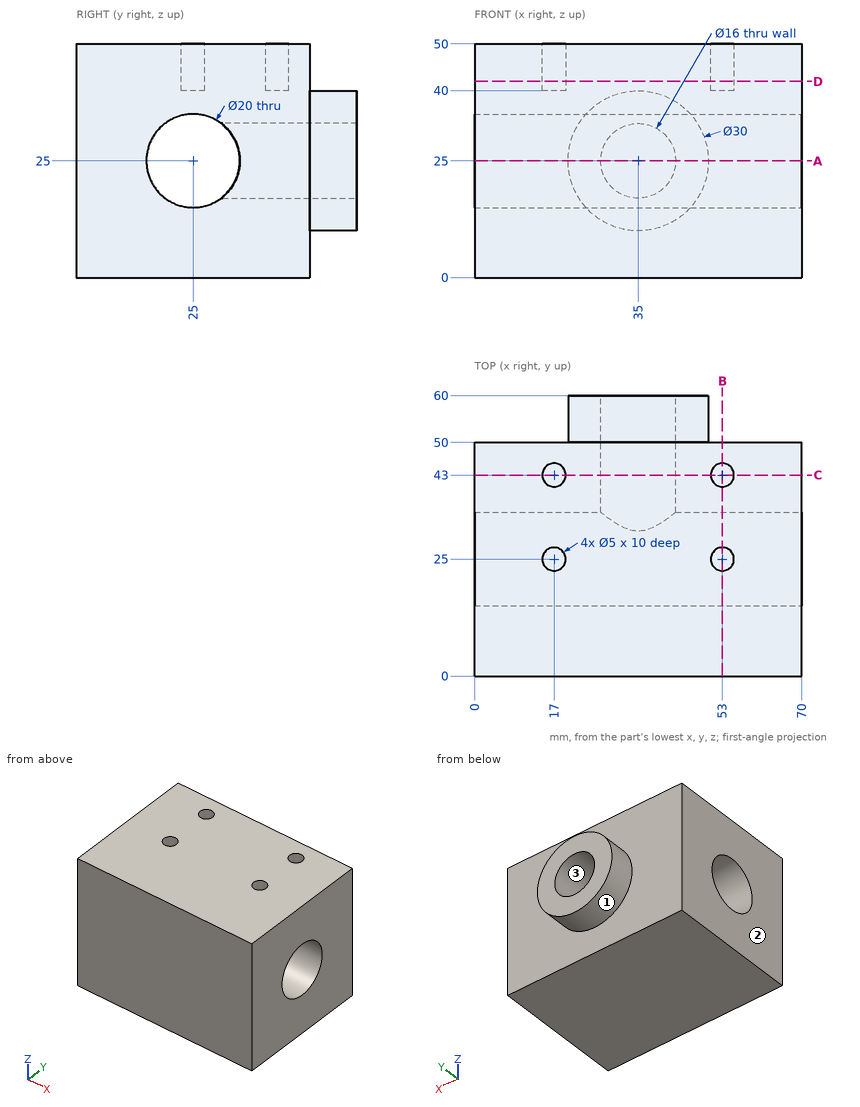
Study the drawing (mm; zero at the part's minimum x, y, z) and answer. Give positions to 0.01 mm unless a question says otherwise; leave off trailing zeros. Order: outer loops, then holes, each group sorted by start corner. A loop starts at its lowest first (then second) coordinate and runs counter-clockwise, first axis right, second up. Notation, with made-up numbers: (49.25, 31) -> (97.25, 31) arc R4 cw to (97.25, 37) -> close; hole circle Ø8 at (16, 45). An arc over 180 degrees is marked (long way). Write item = value, one per line.
1. Given pin 1 (2.5 mm diameter, centred on x = 17.5, y = 43.5, fed in from +Z); pin 2 (1.5 mm diameter, centred on x = 34, z = 31, fed in from +Y); pin 3 (5 mm diameter, centred on y = 53.5, z = 29, fed in from +X), each flat-ended and moving along its own axis, determine where each tip first touches the part or whether it passes through.
Numbers:
pin_1 = 40
pin_2 = 17.62
pin_3 = 49.92
2. The mould has two halves that part along Z. Classify the marked faces 1, 2 and 3: +Z half, -Z half, draft (parallel to the pull), parting line (faces both ways), or undercut.
Numbers:
face_1 = parting line
face_2 = draft
face_3 = undercut
3. A cutting plane is placed at C-C, the plane y = 43. Write down the section's boundary in (x, z).
Numbers:
outline = (0, 0) -> (70, 0) -> (70, 50) -> (55.5, 50) -> (55.5, 40) -> (50.5, 40) -> (50.5, 50) -> (19.5, 50) -> (19.5, 40) -> (14.5, 40) -> (14.5, 50) -> (0, 50) -> close; hole circle Ø16 at (35, 25)
4. A cutting plane is placed at B-B, the plane x = 53. Write down the section's boundary in (y, z), and give its area (3 significant figures).
Numbers:
outline = (0, 0) -> (50, 0) -> (50, 50) -> (45.5, 50) -> (45.5, 40) -> (40.5, 40) -> (40.5, 50) -> (27.5, 50) -> (27.5, 40) -> (22.5, 40) -> (22.5, 50) -> (0, 50) -> close; hole circle Ø20 at (25, 25)
area = 2,090 mm²
5. Straight lines are drawn through the part: line 1 along Y through (x, z) = (53, 44.5); line 2 along Y through (x, z) = (53, 25); line 3 along Z through (x, y) = (5.5, 19). For each, find the intervals that lie inside material, in ascending order.
Numbers:
line_1 = 0 to 22.5, 27.5 to 40.5, 45.5 to 50
line_2 = 0 to 15, 35 to 50
line_3 = 0 to 17, 33 to 50
6. A cutting plane is placed at A-A, the plane z = 25. Write down the section's boundary in (x, y), and give its area (3 significant figures).
Numbers:
outline = (0, 0) -> (70, 0) -> (70, 15) -> (0, 15) -> close; (0, 35) -> (27, 35) -> (27, 60) -> (20, 60) -> (20, 50) -> (0, 50) -> close; (43, 35) -> (70, 35) -> (70, 50) -> (50, 50) -> (50, 60) -> (43, 60) -> close
area = 2,000 mm²
7. A cutting plane is placed at D-D, the plane z = 42. Write down the section's boundary in (x, y), and give its area (3 significant figures).
Numbers:
outline = (0, 0) -> (70, 0) -> (70, 50) -> (0, 50) -> close; hole circle Ø5 at (17, 25); hole circle Ø5 at (17, 43); hole circle Ø5 at (53, 25); hole circle Ø5 at (53, 43)
area = 3,420 mm²
